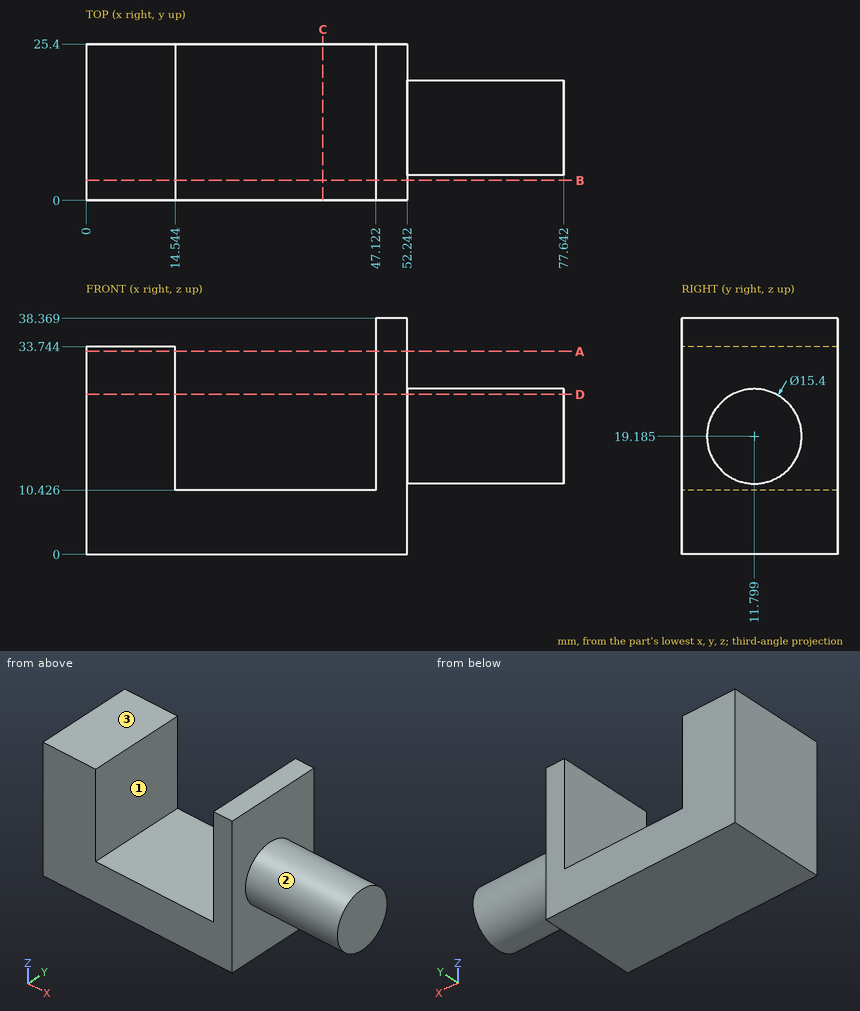
Input: dimensioned drawing with shaded views. Units: mm. Origin: part minimum x, y, z. A direction names the side the tool comes from. Coordinates: 2 decimals unless noted, no trailing zeros. Loops run counter-clockwise (first coordinate to the right, second up) from the corner with the lowest first, then second, coordinate; pieces in that order, holes last. Notation, with made-up numbers: (23.5, -31.5) -> (74.5, -31.5) arc R29 ccw to (74.5, -10.5) -> close; hole circle Ø10 at (57, 74). An arc over 180 degrees is marked (long way). One line per item, written item: value. Start each with the question number.
Q1. Section query D-D, the plane z = 26. Return the cut outline in (x, y).
Q2. Section query A-A, the plane z = 33. Return the cut outline in (x, y).
Q3. Contact query for flat-ended pins moving along their axis: P1, Ø1, axis at y = 22, z = 7.5, coming from the +X side; P2, Ø1.5, axis at x = 58.5, y = 9, coming from the +Z side; P3, Ø7.5, axis at x = 33, y = 11, coming from the +Z side. Output: stop coordinate, or through.
Q4. Section query C-C, the plane x = 38.5. Return the cut outline in (y, z) (1 decimal), and give its area (3 significant figures).
Q5. Section query B-B, the plane y = 3.25. Return the cut outline in (x, z) (1 decimal).
Q6. Set-up query: the marked faces 1, 2 and 3. Return all of +Z, -Z, +X, -X, +Y, -Y with unobstructed straight access to the full face (end or side cutting, diameter ignored); none if empty.
Q7. Line query: line 1 along X through (y, z) = (22.25, 14.5); line 2 along X through (y, z) = (8.5, 23); line 3 along Z through (x, y) = (21.5, 13.75) (1 decimal). Output: solid intervals per line, ascending.
Results:
1. outline: (0, 0) -> (14.54, 0) -> (14.54, 25.4) -> (0, 25.4) -> close; (47.12, 0) -> (52.24, 0) -> (52.24, 8.22) -> (77.64, 8.22) -> (77.64, 15.38) -> (52.24, 15.38) -> (52.24, 25.4) -> (47.12, 25.4) -> close
2. outline: (0, 0) -> (14.54, 0) -> (14.54, 25.4) -> (0, 25.4) -> close; (47.12, 0) -> (52.24, 0) -> (52.24, 25.4) -> (47.12, 25.4) -> close
3. P1: x = 52.24
3. P2: z = 26.61
3. P3: z = 10.43
4. outline: (0, 0) -> (25.4, 0) -> (25.4, 10.4) -> (0, 10.4) -> close
4. area: 265 mm^2
5. outline: (0, 0) -> (52.2, 0) -> (52.2, 38.4) -> (47.1, 38.4) -> (47.1, 10.4) -> (14.5, 10.4) -> (14.5, 33.7) -> (0, 33.7) -> close
6. face 1: +Z, +Y, -Y
6. face 2: +X
6. face 3: +Z, -X, +Y, -Y
7. line 1: 0 to 14.54, 47.12 to 52.24
7. line 2: 0 to 14.54, 47.12 to 77.64
7. line 3: 0 to 10.4
